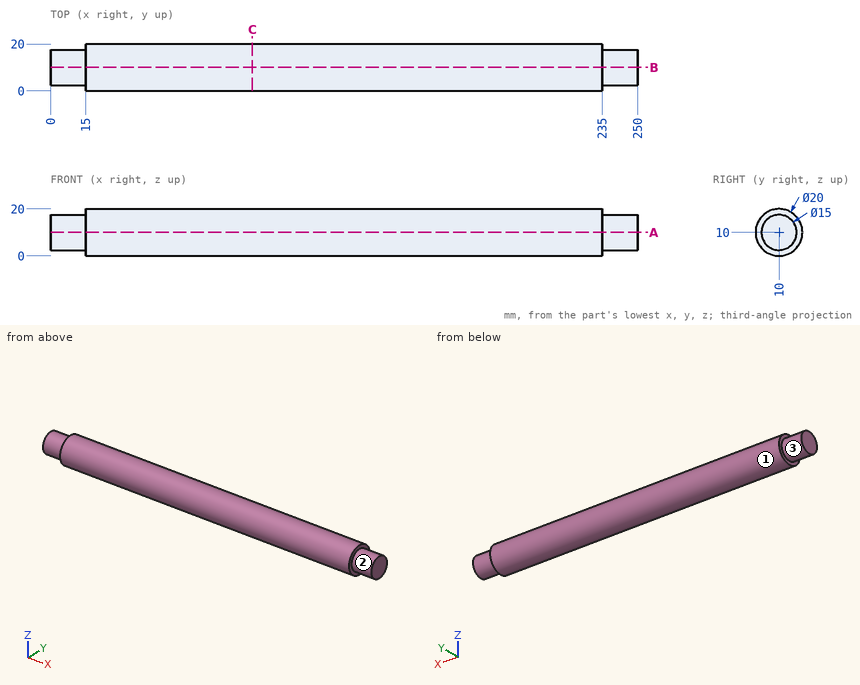
Design review of the part shown in the three views and the two pictorial views. Dimensions are in mm from the part's minimum x, y and z. A direction names the side the tool comes from. Round coordinates to 2 decimals unless told otherwise and drop trailing zeros. Loops run counter-clockwise (first coordinate to the right, second up) from the corner with the lowest first, then second, coordinate; pieces in that order, holes last. Notation, with made-up numbers: M 75.5,11 L 93.5,11 A13 cw 93.5,20 Z; hole C 53,-16 d4. An arc over 180 degrees is marked long. Write item = value, one per line.
Item 1: For line 1 (X direction, y = 2.5, z = 7.5); line 2 (Z direction, x = 229, y = 9.5); line 3 (Y direction, x = 30, z = 10.75), list the stretches that pass through material, from the lowest coordinate up. Write a range as [from, to].
Return value:
line_1 = [15, 235]
line_2 = [0.01, 19.99]
line_3 = [0.03, 19.97]
Item 2: Machinability: for the marked faces 1, 2 and 3, which of the approach directions +Z, -Z, +X, -X, +Y, -Y give a long, thin tool a straight path to every point of the face, cutting with its end or side? Answer none if there is none.
Return value:
face_1 = +X, -X
face_2 = +X
face_3 = -X
Item 3: Take a section at C-C on x = 86. Write out the cut boundary in (y, z), then the cut area to 3 significant figures.
Return value:
outline = C 10,10 d20
area = 314 mm2
Item 4: Insertion check: P1, Ø8, axis at x = 73.5, y = 16, coming from the -Z side; P2, Ø3, axis at x = 44.5, z = 6, coming from the -Y side; P3, Ø2, axis at x = 53, y = 3.5, coming from the +Z side. Each pin has a flat end and moves straight along its axis. Give the tip position at first contact, or say it passes through.
Return value:
P1 = 0.2
P2 = 0.32
P3 = 18.35
Item 5: Take a section at A-A on z = 10. Write out the cut boundary in (x, y).
Return value:
outline = M 0,2.5 L 15,2.5 L 15,0 L 235,0 L 235,2.5 L 250,2.5 L 250,17.5 L 235,17.5 L 235,20 L 15,20 L 15,17.5 L 0,17.5 Z
